The drawing under review shows one solid part. Ordinate dimensions are in mm from its lowest x, y, z. A direction names the side the tool comes from. Give positions to 0.01 mm unless a question says otherwise; leave off trailing zeros. Loops run counter-clockwise (first coordinate to the right, second up) from the corner with the lowest first, then second, coordinate; pieces in that order, holes last. Notation, with made-up numbers: (72.25, 47) - (96.25, 47) arc R14 ccw to (96.25, 55) - close; hole circle Ø8 at (-24, 56). An arc over 180 degrees is marked (long way). Answer as CSV lines item,"result".
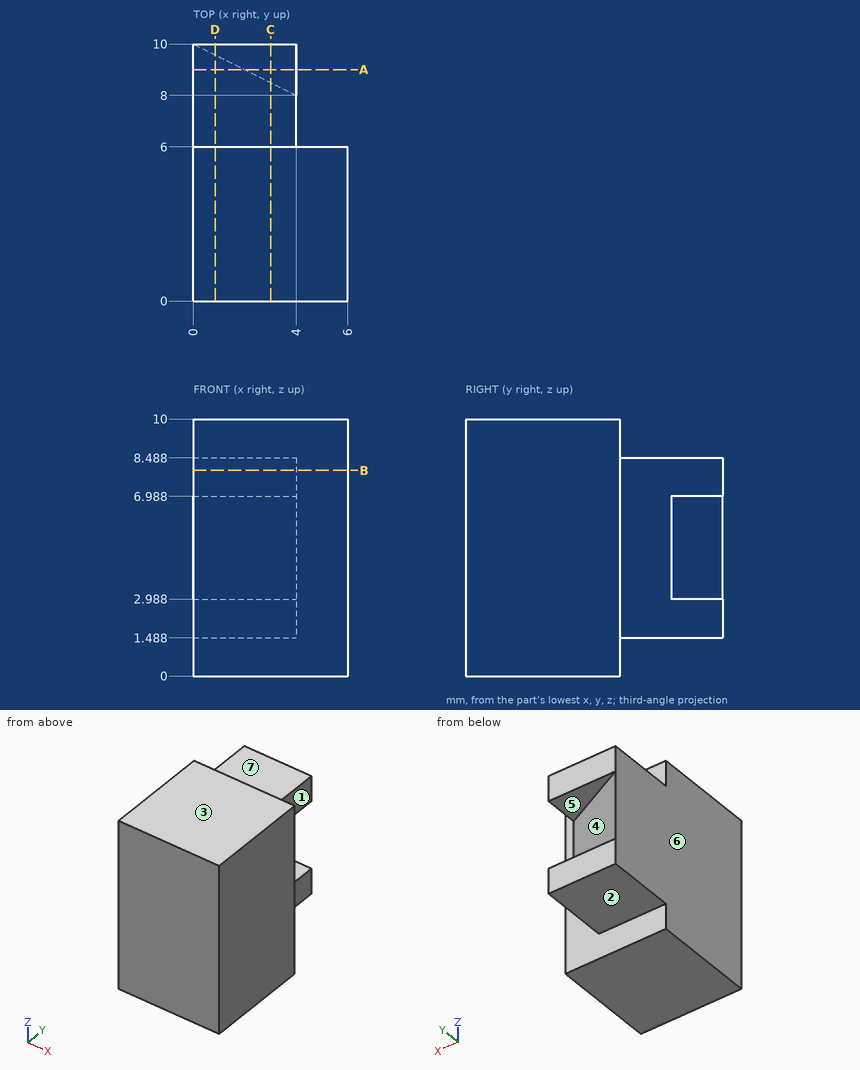
1) Consider section D-D on x = 0.85. Write out the cut boundary in (y, z) (1 decimal).
From the geometry:
outline,"(0, 0) - (6, 0) - (6, 1.5) - (10, 1.5) - (10, 3) - (9.6, 3) - (9.6, 7) - (10, 7) - (10, 8.5) - (6, 8.5) - (6, 10) - (0, 10) - close"
2) Wall thickness on line 1 (Z direction, x = 3.5, y = 8.75); line 2 (X direction, y = 8.75, z = 1.75); line 3 (Z direction, x = 1.8, y = 7.5): over which ranges is each line inside the solid? List them lowest first. Write a range as from..to.
From the geometry:
line 1,"z = 1.49..2.99, 6.99..8.49"
line 2,"x = 0..4"
line 3,"z = 1.49..8.49"
3) Consider section A-A on y = 9. Write out the cut boundary in (x, z).
From the geometry:
outline,"(0, 1.49) - (4, 1.49) - (4, 2.99) - (2, 2.99) - (2, 6.99) - (4, 6.99) - (4, 8.49) - (0, 8.49) - close"
4) Consider section C-C on x = 3. Write out the cut boundary in (y, z), and give its area (3 significant figures).
From the geometry:
outline,"(0, 0) - (6, 0) - (6, 1.49) - (10, 1.49) - (10, 2.99) - (8.5, 2.99) - (8.5, 6.99) - (10, 6.99) - (10, 8.49) - (6, 8.49) - (6, 10) - (0, 10) - close"
area,"82.0 mm^2"
5) Consider section B-B on z = 8. Write out the cut boundary in (x, y).
From the geometry:
outline,"(0, 0) - (6, 0) - (6, 6) - (4, 6) - (4, 10) - (0, 10) - close"
6) Draft analysis for pull direction Z (two halves, no side actions). For the marked faces 5, 6 and 7, state which applies: pulls with the +Z half, pulls with the -Z half, needs draft (parallel to the pull), parting line crosses it, or undercut.
From the geometry:
face 5,"undercut"
face 6,"needs draft"
face 7,"pulls with the +Z half"
7) Machinability: for the marked faces 1, 2, 3 and 4, which of the approach directions +Z, -Z, +X, -X, +Y, -Y give a long, thin tool a straight path to every point of the face, cutting with its end or side? Answer none if there is none.
From the geometry:
face 1,"+Z, -Z, +X, +Y"
face 2,"-Z, +X, -X, +Y"
face 3,"+Z, +X, -X, +Y, -Y"
face 4,"+X, +Y"
8) Insertion check: P1, Ø3, axis at x = 2.5, y = 8.5, coming from the -Z side; P2, Ø3, axis at x = 1.5, y = 8.5, coming from the +Z side; P3, Ø1.2, axis at y = 9, z = 5.5, coming from the +X side. Each pin has a flat end and moves straight along its axis. Give the tip position at first contact, or say it passes through.
From the geometry:
P1,"stops at z = 1.49"
P2,"stops at z = 8.49"
P3,"stops at x = 3.2"
